Check sheet for the drawn part. Datum: minimum x, y, z corner. Units: mm. A direction names the side the tool comes from. Coordinates: 2 decimals unless noted, no trailing zeros. Order: outer loops, then holes, each group sorted by start corner. A loop starts at its lowest first (then second) coordinate and runs counter-clockwise, first axis right, second up. Notation, with made-up numbers: M -24.5,12 L -3.5,12 A24 ccw -3.5,25 Z; hole C 7.25,36 d3. An arc over 180 degrees is marked long. Answer in a Markdown table with one row per item. Add a question column.
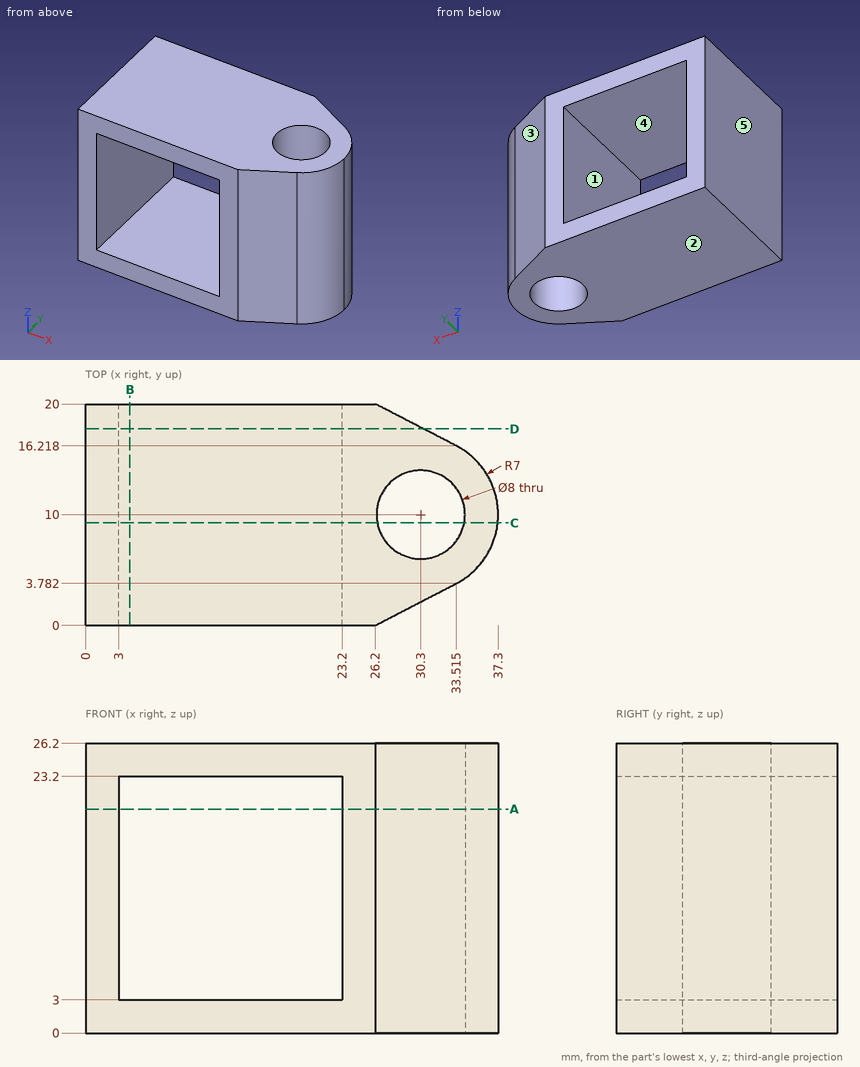
1. Section check A-A on z = 20.25. Enter the section's corners in (x, y) (3 decimals), then the cut area to 3 significant figures.
2. Section check C-C on y = 9.25. Enter the section's corners in (x, z), then the cut area to 3 significant figures.
3. Scan lines: line 1 (Z direction, x = 22, y = 3.75); line 2 (X direction, y = 11.5, z = 19.25); line 3 (X direction, y = 11, z = 21.5). Record each from-to range of solid material in increasing order.
4. Release check for a two-part mould opening along X. For the marked faces 3, 4 and 5 record: released by +X, released by -X, zero draft, split by the parting line, or undercut.
5. Go/stop test with a flat-tipped pin: pin 1 Ø1 at (x, y) = (30, 13) entering from +Z. Record where the tip stops, or that it passes through.
6. Section check B-B on x = 4. Enter the section's corners in (y, z), then the cut area to 3 significant figures.
7. Section check D-D on y = 17.75. Enter the section's corners in (x, z).
8. Set-up check for the marked faces 1 and 2: record each of +Z, -Z, +X, -X, +Y, -Y from which the full face is reachable in a straight line by a thin tool's end or side.
Result sheet:
| question | item | result |
|---|---|---|
| 1 | outline | M 0,0 L 3,0 L 3,20 L 0,20 Z; M 23.2,0 L 26.2,0 L 33.515,3.782 A7 ccw 33.515,16.218 L 26.2,20 L 23.2,20 Z; hole C 30.3,10 d8 |
| 1 | area | 222 mm^2 |
| 2 | outline | M 0,0 L 26.37,0 L 26.37,26.2 L 0,26.2 Z; M 34.23,0 L 37.26,0 L 37.26,26.2 L 34.23,26.2 Z; hole M 3,3 L 23.2,3 L 23.2,23.2 L 3,23.2 Z |
| 2 | area | 362 mm^2 |
| 3 | line 1 | 0 to 3, 23.2 to 26.2 |
| 3 | line 2 | 0 to 3, 23.2 to 26.59, 34.01 to 37.14 |
| 3 | line 3 | 0 to 3, 23.2 to 26.43, 34.17 to 37.23 |
| 4 | face 3 | released by +X |
| 4 | face 4 | undercut |
| 4 | face 5 | released by -X |
| 5 | pin 1 | through |
| 6 | outline | M 0,0 L 20,0 L 20,3 L 0,3 Z; M 0,23.2 L 20,23.2 L 20,26.2 L 0,26.2 Z |
| 6 | area | 120 mm^2 |
| 7 | outline | M 0,0 L 30.55,0 L 30.55,26.2 L 0,26.2 Z; hole M 3,3 L 23.2,3 L 23.2,23.2 L 3,23.2 Z |
| 8 | face 1 | +Y, -Y |
| 8 | face 2 | -Z, +X, -X, +Y, -Y |
